Model file for the job. Use its own axes, mm. Face numbers are marked on the shaded views. A direction names the side the tool comes from. Coordinates: 2 decimals unless noted, no trailing zeros. Write each loop counter-clockwise with the first axis right and the second up, starting at its lowest first coordinate (ties: lowest second). Pieces come first, ordered by that corner, then holes. Notation, with made-up numbers: M 48,-28 L 99,-28 A30 ccw 99,10 Z; hole C 45.5,16 d9. An arc over 180 degrees is marked long. One line per question, with ' | ' between items. Start each with the question number.
(1) Cut at D-D (y = -102). Write the cut outline in (x, z), plus the area to 3 significant figures.
(2) Wall check: probe 1 along Z at (x, y) = (9, 30); probe 2 along X at (y, z) = (-8, -31.5); probe 3 along X at (y, z) = (11, -3). Give the ranges that are in metal, low to high.
(3) Cut at A-A (x = 4). Write the cut outline in (y, z), plus the area to 3 significant figures.
(4) Flat gauge pins, fed straight in: pin 1 Ø12 at (y, z) = (-34, -29.5) entering from -X; pin 2 Ø2 at (x, z) = (63.5, -26) entering from -Y; pin 3 Ø2 at (y, z) = (-29.5, -17) entering from -X. Where does each tip first touch, or does it go through?
(5) Cut at B-B (z = -20). Write the cut outline in (x, y).
(6) Cut at C-C (y = -10). Write the cut outline in (x, z).
(7) Tool access for the marked faces 1 and 2: list every direction of +Z, -Z, +X, -X, +Y, -Y with a clear straight run to the whole face (end or side of a thin tool).
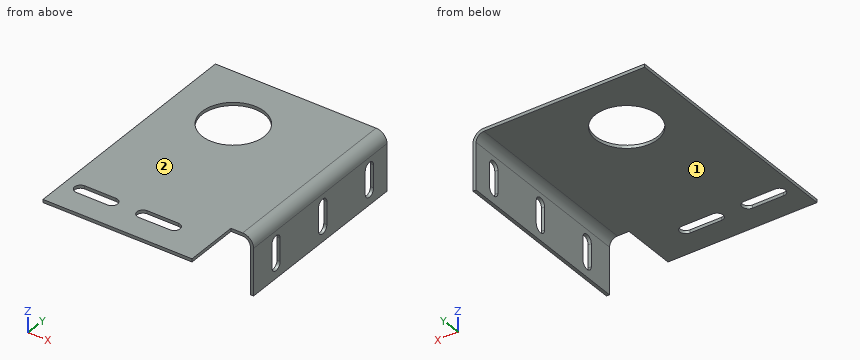
from build123d import *

# Parameters (mm, degrees)
SKETCH1_W                    = 139.7
SKETCH1_H                    = 152.4
SKETCH1_R                    = 25.4
BOSS_EXTRUDE1_DEPTH          = 2.54
EDGE_FLANGE1_STRIP_W         = 22.86
EDGE_FLANGE1_STRIP_H         = 2.54
EDGE_FLANGE1_STRIP_CUT_DEPTH = 152.4
EDGE_FLANGE1_DEPTH           = 152.4
CUT_EXTRUDE3_DEPTH           = 2.54
SKETCH10_W                   = 121.292072418
SKETCH10_H                   = 2.54
BOSS_EXTRUDE2_DEPTH          = 44.45
CUT_EXTRUDE2_DEPTH           = 44.45


# Sheet-metal steps are written as plain solids
with BuildPart() as part:
    # Sketch1 → Boss-Extrude1 (new body)
    with BuildSketch(Plane.XY):
        with Locations((-5.388148668, -29.389901823)):
            Rectangle(SKETCH1_W, SKETCH1_H)
        with Locations((-24.438148668, -3.989901823)):
            Circle(SKETCH1_R, mode=Mode.SUBTRACT)
    extrude(amount=BOSS_EXTRUDE1_DEPTH)

    # Edge-Flange1 strip (across the edge) → Edge-Flange1 strip cut (cut)
    with BuildSketch(Plane(origin=(64.461851332, 46.810098177, 0), x_dir=(-1, 0, 0), z_dir=(0, -1, 0))):
        with Locations((-2.54, -1.27)):
            Rectangle(EDGE_FLANGE1_STRIP_W, EDGE_FLANGE1_STRIP_H)
    extrude(amount=EDGE_FLANGE1_STRIP_CUT_DEPTH, mode=Mode.SUBTRACT)

    # Edge-Flange1 section (across the edge) → Edge-Flange1 (add)
    with BuildSketch(Plane(origin=(64.461851332, 46.810098177, 0), x_dir=(-1, 0, 0), z_dir=(0, -1, 0))):
        with BuildLine():
            Line((0, 6.35), (0, 44.45))
            Line((0, 44.45), (2.54, 44.45))
            Line((2.54, 44.45), (2.54, 6.35))
            ThreePointArc((2.54, 6.35), (4.399871939, 1.859871939), (8.89, 0))
            Line((8.89, 0), (8.89, -2.54))
            ThreePointArc((8.89, -2.54), (2.603820715, 0.063820715), (0, 6.35))
        make_face()
    extrude(amount=EDGE_FLANGE1_DEPTH)

    # Sketch9 → Cut-Extrude3 (cut)
    with BuildSketch(Plane.ZY.offset(-61.921851332)):
        with BuildLine():
            Line((-14.954545697, 31.473568276), (-33.436292004, 31.473568276))
            ThreePointArc((-33.436292004, 31.473568276), (-38.198792004, 26.711068276), (-33.436292004, 21.948568276))
            Line((-33.436292004, 21.948568276), (-14.954545697, 21.948568276))
            ThreePointArc((-14.954545697, 21.948568276), (-10.192045697, 26.711068276), (-14.954545697, 31.473568276))
        make_face()
        with BuildLine():
            Line((-14.954545697, -21.866431724), (-33.436292004, -21.866431724))
            ThreePointArc((-33.436292004, -21.866431724), (-38.198792004, -26.628931724), (-33.436292004, -31.391431724))
            Line((-33.436292004, -31.391431724), (-14.954545697, -31.391431724))
            ThreePointArc((-14.954545697, -31.391431724), (-10.192045697, -26.628931724), (-14.954545697, -21.866431724))
        make_face()
        with BuildLine():
            Line((-14.954545697, -75.206431724), (-33.436292004, -75.206431724))
            ThreePointArc((-33.436292004, -75.206431724), (-38.198792004, -79.968931724), (-33.436292004, -84.731431724))
            Line((-33.436292004, -84.731431724), (-14.954545697, -84.731431724))
            ThreePointArc((-14.954545697, -84.731431724), (-10.192045697, -79.968931724), (-14.954545697, -75.206431724))
        make_face()
    extrude(amount=-CUT_EXTRUDE3_DEPTH, mode=Mode.SUBTRACT)

    # Sketch10 → Boss-Extrude2 (add)
    with BuildSketch(Plane.XZ.offset(105.589901823)):
        with Locations((-14.592112459, 1.27)):
            Rectangle(SKETCH10_W, SKETCH10_H)
    extrude(amount=BOSS_EXTRUDE2_DEPTH)

    # Sketch11 → Cut-Extrude2 (cut)
    with BuildSketch(Plane.XY.offset(2.54)):
        with BuildLine():
            Line((-62.024050091, -120.904110835), (-36.624050091, -120.904110835))
            ThreePointArc((-36.624050091, -120.904110835), (-31.798050091, -125.730110835), (-36.624050091, -130.556110835))
            Line((-36.624050091, -130.556110835), (-62.024050091, -130.556110835))
            ThreePointArc((-62.024050091, -130.556110835), (-66.850050091, -125.730110835), (-62.024050091, -120.904110835))
        make_face()
        with BuildLine():
            Line((-11.224050091, -120.904110835), (14.175949909, -120.904110835))
            ThreePointArc((14.175949909, -120.904110835), (19.001949909, -125.730110835), (14.175949909, -130.556110835))
            Line((14.175949909, -130.556110835), (-11.224050091, -130.556110835))
            ThreePointArc((-11.224050091, -130.556110835), (-16.050050091, -125.730110835), (-11.224050091, -120.904110835))
        make_face()
    extrude(amount=-CUT_EXTRUDE2_DEPTH, mode=Mode.SUBTRACT)


solid = part.part
Filled in:
1) outline: M -75.24,0 L 55.57,0 A6.35 cw 61.92,-6.35 L 61.92,-44.45 L 64.46,-44.45 L 64.46,-6.35 A8.89 ccw 55.57,2.54 L -75.24,2.54 Z | area: 459 mm²
2) probe 1: 0 to 2.54 | probe 2: 61.92 to 64.46 | probe 3: 60.97 to 63.81
3) outline: M -150.04,0 L -130.56,0 L -130.56,2.54 L -150.04,2.54 Z; M -120.9,0 L 46.81,0 L 46.81,2.54 L -120.9,2.54 Z | area: 475 mm²
4) pin 1: x = 61.92 | pin 2: y = -105.59 | pin 3: through
5) outline: M 61.92,-105.59 L 64.46,-105.59 L 64.46,-84.73 L 61.92,-84.73 Z; M 61.92,-75.21 L 64.46,-75.21 L 64.46,-31.39 L 61.92,-31.39 Z; M 61.92,-21.87 L 64.46,-21.87 L 64.46,21.95 L 61.92,21.95 Z; M 61.92,31.47 L 64.46,31.47 L 64.46,46.81 L 61.92,46.81 Z
6) outline: M -75.24,0 L -49.12,0 L -49.12,2.54 L -75.24,2.54 Z; M 0.24,0 L 55.57,0 A6.35 cw 61.92,-6.35 L 61.92,-44.45 L 64.46,-44.45 L 64.46,-6.35 A8.89 ccw 55.57,2.54 L 0.24,2.54 Z
7) face 1: -Z, -X, +Y, -Y | face 2: +Z, +X, -X, +Y, -Y
